Autodesk Inventor part; units mm, degrees
ref_plane "YZ Plane" through (0, 0, 0) normal (1, 0, 0) x (0, 1, 0)
ref_plane "XZ Plane" through (0, 0, 0) normal (0, 1, 0) x (-1, 0, 0)
ref_plane "XY Plane" through (0, 0, 0) normal (0, 0, 1) x (1, 0, 0)
sketch "Szkic2" plane through (0, 0, 0) normal (0, 0, 1) x (1, 0, 0)
  line L0 (-44, 25) -> (51, 25)
  line L1 (-44, -25) -> (51, -25)
  line L2 (51, -25) -> (51, -6.25)
  line L3 (51, -6.25) -> (26, -6.25)
  line L4 (26, -6.25) -> (26, 6.25)
  line L5 (26, 6.25) -> (51, 6.25)
  line L6 (51, 6.25) -> (51, 25)
  line L7 (-44, -25) -> (-44, -4)
  line L8 (-44, -4) -> (-26, -4)
  line L9 (-26, -4) -> (-26, 4)
  line L10 (-26, 4) -> (-44, 4)
  line L11 (-44, 4) -> (-44, 25)
  line L12 (0, 35) -> (0, -35)
  line L13 (-63, 0) -> (70, 0)
  point P0 (0, 0)
  dimension "d7" = 95
  dimension "d8" = 25
  dimension "d9" = 12.5
  dimension "d10" = 18
  dimension "d11" = 50
  dimension "d12" = 8
extrude "Wyciągnięcie proste1" add sketch "Szkic2" along normal blind 18
sketch "Szkic3" plane through (-44, -25, 0) normal (0, -1, 0) x (1, 0, 0)
  line L0 (0, 0) -> (95, 0)
  line L1 (95, 0) -> (95, 18)
  line L2 (0, 18) -> (95, 18)
  line L3 (0, 0) -> (0, 18)
  circle A0 centre (8, 8.5) radius 4
  circle A1 centre (83, 11) radius 4
  circle A2 centre (43, 18.5) radius 10
  point P0 (44, 0)
  dimension "d16" = 11
  dimension "d19" = 9.5
  dimension "d21" = 20
  dimension "d22" = 43
  dimension "d23" = 40
  dimension "d24" = 35
  dimension "d25" = 8
  dimension "d26" = 0.5
  dimension "d27" = 8
extrude "Wyciągnięcie proste2" cut sketch "Szkic3" against normal through all contours A2 L2 | L2 A2 | A0 | A1
sketch "Szkic4" plane through (0, 0, 18) normal (0, 0, 1) x (1, 0, 0)
  line L0 (0, 35) -> (0, -35)
  line L1 (-63, 0) -> (70, 0)
  point P0 (0, 0)
  point P1 (21, -12.3158)
  point P2 (21, 17.6842)
  point P3 (-21, 17.6842)
  point P4 (-21, -12.3158)
  dimension "d30" = 42
  dimension "d31" = 30
hole "Otwór1" at (21, -12.3158, 18) at (21, 17.6842, 18) at (-21, 17.6842, 18) at (-21, -12.3158, 18) direction (0, 0, -1) diameter 9 depth 20 tip angle 118 counterbore diameter 14 counterbore depth 6
properties part number "Podstawa"
Source: CAD feature listing. Evaluate the final solid. Frame: model axes, mm. A direction names the side the tool comes from. Round coordinates to 2 decimals unless told otherwise and drop trailing zeros. Loops run counter-clockwise (first coordinate to the right, second up) from the corner with the lowest first, then second, coordinate; pieces in that order, holes last. Notation, with made-up numbers: M 17.25,49 L 72.25,49 A17 cw 72.25,72 Z; hole C -24.75,13 d3. An arc over 180 degrees is marked long. Use a Markdown table: item, result. Add a question column.
1. Cut plane A-A, the plane x = 39. Output: boundary loops of the cut face in (y, z).
2. Cut plane D-D, the plane y = -21. Output: boundary loops of the cut face in (x, z), and give its area (3 significant figures).
3. Contact query for flat-ended pins moving along their axis: pin 1 (6.5 mm diameter, centred on y = 0, z = 5.5, fed in from -X); pin 2 (11.5 mm diameter, centred on x = 21, y = 17.68, fed in from +Z); pin 3 (8 mm diameter, centred on x = 0.5, y = -7, fed in from +Z). Output: stop coordinate, or through.
4. Ray query, line 1 along Y through (x, z) = (21, 16.25); line 2 along Y through (x, z) = (21, 7); line 3 along Y through (x, z) = (-35.5, 16.5). Return the intervals inside material, ascending. Write a range as [from, to].
5. Cut plane B-B, the plane y = 16. Output: boundary loops of the cut face in (x, z), and give its area (3 significant figures).
6. Cut plane C-C, the plane x = 21. Output: boundary loops of the cut face in (y, z), and give its area (3 significant figures).
7. Pull-direction query (Y, two-part tool) for faces 6 (the flat face through (26, 18, 12)), 7 (the flat face through (25, 0, 18)); classes: +Y half, -Y half, draft (parallel to the pull), parting line (faces both ways), or undercut.
8. Set-up query: faces 1 (the flat face through (-44, 14, 9)), 2 (the flat face through (-16, -12, 12)), 3 (the flat face through (-26, 0, 9)), 4 (the flat face through (51, -16, 9)), 5 (the flat face through (38.3, 6.25, 6.9)). Return all of +Z, -Z, +X, -X, +Y, -Y with unobstructed straight access to the full face (end or side cutting, diameter ignored); none if empty.
Solution:
| question | item | result |
|---|---|---|
| 1 | outline | M -25,0 L -6.25,0 L -6.25,7 L -25,7 Z; M -25,15 L -6.25,15 L -6.25,18 L -25,18 Z; M 6.25,0 L 25,0 L 25,7 L 6.25,7 Z; M 6.25,15 L 25,15 L 25,18 L 6.25,18 Z |
| 2 | outline | M -44,0 L 51,0 L 51,18 L 8.99,18 A10 cw -10.99,18 L -44,18 Z; hole C -36,8.5 d8; hole C 39,11 d8 |
| 2 | area | 1,460 mm2 |
| 3 | pin 1 | stops at x = -26 |
| 3 | pin 2 | stops at z = 12 |
| 3 | pin 3 | stops at z = 10.15 |
| 4 | line 1 | y = [-25, -19.32], [-5.32, 10.68], [24.68, 25] |
| 4 | line 2 | y = [-25, -16.82], [-7.82, 13.18], [22.18, 25] |
| 4 | line 3 | y = [-25, -4], [4, 25] |
| 5 | outline | M -44,0 L -25.17,0 L -25.17,12 L -27.79,12 L -27.79,18 L -44,18 Z; M -16.83,0 L 16.83,0 L 16.83,12 L 14.21,12 L 14.21,18 L 8.99,18 A10 cw -10.99,18 L -14.21,18 L -14.21,12 L -16.83,12 Z; M 25.17,0 L 51,0 L 51,18 L 27.79,18 L 27.79,12 L 25.17,12 Z; hole C -36,8.5 d8; hole C 39,11 d8 |
| 5 | area | 1,100 mm2 |
| 6 | outline | M -25,0 L -16.82,0 L -16.82,12 L -19.32,12 L -19.32,18 L -25,18 Z; M -7.82,0 L 13.18,0 L 13.18,12 L 10.68,12 L 10.68,18 L -5.32,18 L -5.32,12 L -7.82,12 Z; M 22.18,0 L 25,0 L 25,18 L 24.68,18 L 24.68,12 L 22.18,12 Z |
| 6 | area | 516 mm2 |
| 7 | face 6 | undercut |
| 7 | face 7 | draft |
| 8 | face 1 | +Z, -Z, -X, +Y, -Y |
| 8 | face 2 | +Z |
| 8 | face 3 | +Z, -Z, -X |
| 8 | face 4 | +Z, -Z, +X, +Y, -Y |
| 8 | face 5 | +Z, -Z, +X |
